Check sheet for the modelled part. Datum: model origin and axes. Units: mm. Round coordinates to 2 decimals unless told otherwise and drop trailing zeros. Order: outer loops, then holes, each group sorted by start corner. A loop starts at its lowest first (then second) coordinate and runs counter-clockwise, first axis right, second up.
Q1. Depth check by flat-ended pin: P1, Ø4, axis at x = 645, z = -368.5, coming from the -Y side; P2, Ø4, axis at x = 814.5, y = 16.5, coming from the +Z side; P3, Ø14, axis at x = 1040, y = -18.5, coming from the -Z side. Enter the tip coordinate at first touch or a pass-through.
Q2. Cross-section at A-A on x = 1104. Record the cut outline in (y, z), then the cut area to 3 significant figures.
Q3. Scan lines: probe 1 along Z at (x, y) = (417.5, 20); probe 2 along Z at (x, y) = (1190, 9.5). Record each from-to range of solid material in increasing order.
from build123d import *

# Parameters (mm, degrees)
BOSS_EXTRUDE1_DEPTH = 1430


with BuildPart() as part:
    # Sketch1 → Boss-Extrude1 (new body)
    with BuildSketch(Plane(origin=(0, 0, 0), x_dir=(0, 0, -1), z_dir=(1, 0, 0))):
        with BuildLine():
            Line((360, 25), (-360, 25))
            Line((-360, 25), (-360, 12.5))
            Line((-360, 12.5), (-347.5, 12.5))
            ThreePointArc((-347.5, 12.5), (-335, 0), (-347.5, -12.5))
            Line((-347.5, -12.5), (-360, -12.5))
            Line((-360, -12.5), (-360, -25))
            Line((-360, -25), (360, -25))
            Line((360, -25), (360, -12.5))
            Line((360, -12.5), (347.5, -12.5))
            ThreePointArc((347.5, -12.5), (335, 0), (347.5, 12.5))
            Line((347.5, 12.5), (360, 12.5))
            Line((360, 12.5), (360, 25))
        make_face()
        with BuildLine():
            Line((-347.5, 12.5), (-360, 12.5))
            Line((-360, 12.5), (-360, -12.5))
            Line((-360, -12.5), (-347.5, -12.5))
            ThreePointArc((-347.5, -12.5), (-335, 0), (-347.5, 12.5))
        make_face()
        with BuildLine():
            Line((-360, -12.5), (-360, 12.5))
            Line((-360, 12.5), (-372.5, 12.5))
            ThreePointArc((-372.5, 12.5), (-385, 0), (-372.5, -12.5))
            Line((-372.5, -12.5), (-360, -12.5))
        make_face()
        with BuildLine():
            Line((372.5, 12.5), (360, 12.5))
            Line((360, 12.5), (360, -12.5))
            Line((360, -12.5), (372.5, -12.5))
            ThreePointArc((372.5, -12.5), (385, 0), (372.5, 12.5))
        make_face()
        with BuildLine():
            Line((360, -12.5), (360, 12.5))
            Line((360, 12.5), (347.5, 12.5))
            ThreePointArc((347.5, 12.5), (335, 0), (347.5, -12.5))
            Line((347.5, -12.5), (360, -12.5))
        make_face()
    extrude(amount=BOSS_EXTRUDE1_DEPTH)


solid = part.part
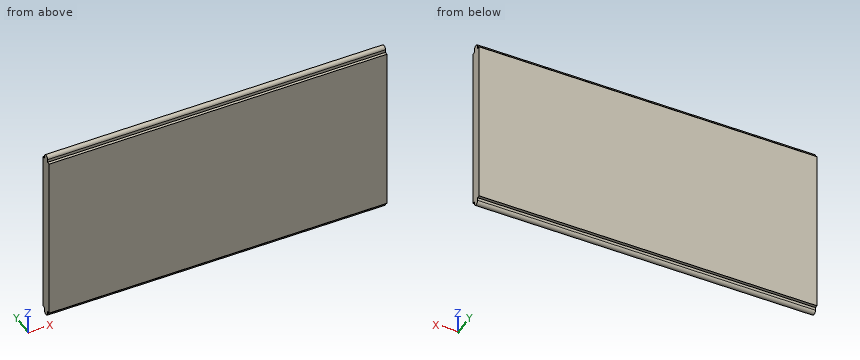
Results found:
1. P1: stops at y = -12.5
1. P2: stops at z = 360
1. P3: stops at z = -377.4
2. outline: (-25, -360) - (-12.5, -360) - (-12.5, -372.5) arc R12.5 ccw to (12.5, -372.5) - (12.5, -360) - (25, -360) - (25, 360) - (12.5, 360) - (12.5, 372.5) arc R12.5 ccw to (-12.5, 372.5) - (-12.5, 360) - (-25, 360) - close
2. area: 37,100 mm2
3. probe 1: z = -360 to 360
3. probe 2: z = -380.62 to 380.62
